Build history of the part. All positions in model axes, mm. A direction names the side the tool comes from. Round coordinates to 2 decimals unless told otherwise and drop trailing zeros. Write each loop counter-clockwise with the first axis right and the second up, starting at its lowest first coordinate (ties: lowest second). Pieces come first, ordered by that corner, then holes. Notation, with made-up numbers: M 6,32.25 L 39,32.25 A33 cw 39,70.25 Z; hole C -7,25 d7. An arc over 180 degrees is marked long. Use a Markdown table: item, result.
from build123d import *

# Parameters (mm, degrees)
SKETCH1_R           = 14.2748
SKETCH1_R_2         = 2.032
BOSS_EXTRUDE1_DEPTH = 14.478


with BuildPart() as part:
    # Sketch1 → Boss-Extrude1 (new body)
    with BuildSketch(Plane(origin=(0, 0, 0), x_dir=(1, 0, 0), z_dir=(0, 1, 0))):
        with Locations(Location((0, 0, 0), (0, 0, 270))):
            Circle(SKETCH1_R)
        with Locations(Location((0, 10.287, 0), (0, 0, 270))):
            Circle(SKETCH1_R_2, mode=Mode.SUBTRACT)
        with Locations(Location((8.908803329, 5.1435, 0), (0, 0, 270))):
            Circle(SKETCH1_R_2, mode=Mode.SUBTRACT)
        with Locations(Location((8.908803329, -5.1435, 0), (0, 0, 270))):
            Circle(SKETCH1_R_2, mode=Mode.SUBTRACT)
        with Locations(Location((0, -10.287, 0), (0, 0, 270))):
            Circle(SKETCH1_R_2, mode=Mode.SUBTRACT)
        with Locations(Location((-8.908803329, -5.1435, 0), (0, 0, 270))):
            Circle(SKETCH1_R_2, mode=Mode.SUBTRACT)
        with Locations(Location((-8.908803329, 5.1435, 0), (0, 0, 270))):
            Circle(SKETCH1_R_2, mode=Mode.SUBTRACT)
        Polygon((7.332348419, 0), (3.666174209, 6.35), (-3.666174209, 6.35), (-7.332348419, 0), (-3.666174209, -6.35), (3.666174209, -6.35), align=None, mode=Mode.SUBTRACT)
    extrude(amount=BOSS_EXTRUDE1_DEPTH)


solid = part.part
Q1. Which spindle directions (+Z, -Z, +X, -X, +Y, -Y) get a long thin tool onto all of the face, cutting with end or side? Do faces 4 (the flat face through (-6, 0, 3)), 5 (the flat face through (0, 7, 6.35)). Say none if no direction does.
Response values:
| item | result |
|---|---|
| face 4 | +Z, -Z, +X, -X, -Y |
| face 5 | +Y, -Y |
Q2. Cut at A-A on x = 0. Give the cut face in (y, z) (3 decimals), and give its area (3 significant figures).
Response values:
| item | result |
|---|---|
| outline | M 0,-14.275 L 14.478,-14.275 L 14.478,-12.319 L 0,-12.319 Z; M 0,-8.255 L 14.478,-8.255 L 14.478,-6.35 L 0,-6.35 Z; M 0,6.35 L 14.478,6.35 L 14.478,8.255 L 0,8.255 Z; M 0,12.319 L 14.478,12.319 L 14.478,14.275 L 0,14.275 Z |
| area | 112 mm2 |
Q3. Cut at B-B on y = 6. Count the separate pieces of the cut face and the enclosed holes in it, and give its area (3 significant figures).
Response values:
| item | result |
|---|---|
| separate pieces | 1 |
| enclosed holes | 7 |
| area | 423 mm2 |
Q4. Drop flat-ended pins along their axis: P1, Ø2, axis at y = 9.5, z = 2.5, coming from the -X side; P2, Ø3.5, axis at x = 8.91, z = -5.14, coming from the -Y side; P3, Ø1.5, axis at y = 5, z = -2, coming from the +X side; P4, Ø8, axis at y = 4.5, z = -9, coming from the +X side. Give the stop position or say it passes through.
Response values:
| item | result |
|---|---|
| P1 | stops at x = -14.2 |
| P2 | passes through |
| P3 | stops at x = 14.22 |
| P4 | stops at x = 13.37 |
Q5. Two-plate mould, pull along X, no slides. Class faces 1 (the cylindrical face through (14.153, 7.138, -1.858)), 2 (the flat face through (-6, 14.478, 3)), 3 (the flat face through (0, 7, -6.35)): +X half, -X half, draft (parallel to the pull), parting line (faces both ways), or undercut.
Response values:
| item | result |
|---|---|
| face 1 | parting line |
| face 2 | draft |
| face 3 | undercut |
Q6. Drill centre lines: L1, parallel to Z at x = -10.25, y = 6.25; L2, parallel to Z at x = -0.75, y = 8; L3, parallel to Z at x = -9.25, y = 8.5. Where is each one in solid material? Low to high.
Response values:
| item | result |
|---|---|
| L1 | z = -9.94 to -6.67, -3.62 to 3.62, 6.67 to 9.94 |
| L2 | z = -14.26 to -12.18, -8.4 to -6.35, 6.35 to 8.4, 12.18 to 14.26 |
| L3 | z = -10.87 to -7.15, -3.14 to 3.14, 7.15 to 10.87 |
Q7. Cut at D-D on z = -10. Give the cut face in (x, y), and give its area (3 significant figures).
Response values:
| item | result |
|---|---|
| outline | M -10.19,0 L -2.01,0 L -2.01,14.48 L -10.19,14.48 Z; M 2.01,0 L 10.19,0 L 10.19,14.48 L 2.01,14.48 Z |
| area | 237 mm2 |
Q8. Cut at C-C on z = 5. Give the cut face in (x, y).
Response values:
| item | result |
|---|---|
| outline | M -13.37,0 L -10.94,0 L -10.94,14.48 L -13.37,14.48 Z; M -6.88,0 L -4.45,0 L -4.45,14.48 L -6.88,14.48 Z; M 4.45,0 L 6.88,0 L 6.88,14.48 L 4.45,14.48 Z; M 10.94,0 L 13.37,0 L 13.37,14.48 L 10.94,14.48 Z |
